```python
from build123d import *

# Parameters (mm, degrees)
SKETCH1_R           = 1.6383
SKETCH1_R_2         = 0.8382
BOSS_EXTRUDE1_DEPTH = 1.575


with BuildPart() as part:
    # Sketch1 → Boss-Extrude1 (new body)
    with BuildSketch(Plane(origin=(0, 0, 0), x_dir=(1, 0, 0), z_dir=(0, 1, 0))):
        with BuildLine():
            Line((-38.39500299, 29.999999735), (-42.73000299, 29.999999735))
            Line((-42.73000299, 29.999999735), (-44.000003042, 30.013999735))
            Line((-44.000003042, 30.013999735), (-44.000003042, 31.269999735))
            Line((-44.000003042, 31.269999735), (-44.00000361, 44.999999735))
            ThreePointArc((-44.00000361, 44.999999735), (-43.414217128, 46.414213903), (-42.000002924, 47.000000297))
            Line((-42.000002924, 47.000000297), (-30.435003745, 47.000000297))
            Line((-30.435003745, 47.000000297), (-30.435002721, 22.255354587))
            Line((-30.435002721, 22.255354587), (-11.909002721, 22.255355354))
            Line((-11.909002721, 22.255355354), (-11.909002721, -8.5))
            Line((-11.909002721, -8.5), (-23.409001447, -8.5))
            Line((-23.409001447, -8.5), (-23.409000495, -31.499999412))
            Line((-23.409000495, -31.499999412), (23.408999505, -31.499997474))
            Line((23.408999505, -31.499997474), (23.408999505, -8.499997555))
            Line((23.408999505, -8.499997555), (11.908997279, -8.499997555))
            Line((11.908997279, -8.499997555), (11.908997279, 22.25535634))
            Line((11.908997279, 22.25535634), (30.434997279, 22.255357107))
            Line((30.434997279, 22.255357107), (30.434996255, 47.000002817))
            Line((30.434996255, 47.000002817), (41.999997246, 47.000002817))
            ThreePointArc((41.999997246, 47.000002817), (43.414210615, 46.414216484), (43.999996958, 45.000003119))
            Line((43.999996958, 45.000003119), (43.999996958, 32.000003378))
            Line((43.999996958, 32.000003378), (43.999996958, 30.014003378))
            Line((43.999996958, 30.014003378), (32.823996958, 30.032002916))
            Line((32.823996958, 30.032002916), (32.823999503, -31.453997084))
            Line((32.823999503, -31.453997084), (36.099999555, -31.453996949))
            Line((36.099999555, -31.453996949), (36.099999785, -36.999996949))
            Line((36.099999785, -36.999996949), (43.849731264, -36.999996949))
            Line((43.849731264, -36.999996949), (43.849731264, -46.999996628))
            Line((43.849731264, -46.999996628), (-42.000000215, -46.999996628))
            ThreePointArc((-42.000000215, -46.999996628), (-43.414212607, -46.414211361), (-44.000000215, -44.999999938))
            Line((-44.000000215, -44.999999938), (-44.000000215, -38.976999938))
            ThreePointArc((-44.000000215, -38.976999938), (-43.409460005, -37.574276579), (-42.000000215, -36.999999938))
            Line((-42.000000215, -36.999999938), (-38.395000215, -36.999999938))
            Line((-38.395000215, -36.999999938), (-36.100000319, -36.999999938))
            Line((-36.100000319, -36.999999938), (-36.100000549, -31.453999938))
            Line((-36.100000549, -31.453999938), (-32.824000497, -31.453999802))
            Line((-32.824000497, -31.453999802), (-32.824003042, 30.014000198))
            Line((-32.824003042, 30.014000198), (-38.39500299, 29.999999735))
        make_face()
        with Locations(Location((40, 43.5, 0), (0, 0, 270))):
            Circle(SKETCH1_R, mode=Mode.SUBTRACT)
        with Locations(Location((-40, 43.5, 0), (0, 0, 270))):
            Circle(SKETCH1_R, mode=Mode.SUBTRACT)
        with Locations(Location((-37.6, -42.2, 0), (0, 0, 270))):
            Circle(SKETCH1_R, mode=Mode.SUBTRACT)
        with Locations(Location((36.1, -42.2, 0), (0, 0, 270))):
            Circle(SKETCH1_R, mode=Mode.SUBTRACT)
        with Locations(Location((-36.785003304, 36.350000034, 0), (0, 0, 270))):
            Circle(SKETCH1_R_2, mode=Mode.SUBTRACT)
        with Locations(Location((-26.220002542, 17.93192918, 0), (0, 0, 270))):
            Circle(SKETCH1_R_2, mode=Mode.SUBTRACT)
        with Locations(Location((26.219997458, 17.931931351, 0), (0, 0, 270))):
            Circle(SKETCH1_R_2, mode=Mode.SUBTRACT)
        with Locations(Location((36.784996695, 36.36800308, 0), (0, 0, 270))):
            Circle(SKETCH1_R_2, mode=Mode.SUBTRACT)
    extrude(amount=BOSS_EXTRUDE1_DEPTH)


solid = part.part
```
Verification items for the finished model (mm, model axes). Give positions to 0.01 mm unless a question says otherwise; leave off trailing zeros. Write each loop counter-clockwise with the first axis right and the second up, starting at its lowest first coordinate (ties: lowest second). Pieces come first, ordered by that corner, then holes. Notation, with made-up numbers: M -13,-22.75 L 32,-22.75 A15 ccw 32,-4.75 Z; hole C 82.25,-4.75 d11. An arc over 180 degrees is marked long. One line per question, with ' | ' between items.
1) Thickness scan on line 1 along X through (y, z) = (0.3, -43.5) (3 decimals); line 2 along X through (y, z) = (0.55, 42.2); line 3 along Z through (x, y) = (-17.5, 1.3). Record the ranges inside material, lowest first. Write a range as [from, to].
Result:
line 1: x = [-44, -41.638], [-38.362, -30.435], [30.435, 38.362], [41.638, 44] | line 2: x = [-44, -39.24], [-35.96, 34.46], [37.74, 43.85] | line 3: z = [-22.26, 8.5], [31.5, 47]
2) Mould release check, pull along X, two halves, no side actions. Record for faces 1 (the cylindrical face through (-43.43, 0.78, -46.4)), 2 (the cylindrical face through (43.4, 0.78, -46.43)), 3 (the cylindrical face through (-39.2, 0.78, 41.84)), 4 (the cylindrical face through (-38.62, 0.78, -42.62)): released by +X, released by -X, zero draft, split by the parting line, or undercut.
Result:
face 1: released by -X | face 2: released by +X | face 3: undercut | face 4: undercut
3) Section check C-C on z = -4.5. Enter the section's corners in (x, y) (3 decimals).
Result:
outline: M -32.824,0 L -11.909,0 L -11.909,1.575 L -32.824,1.575 Z; M 11.909,0 L 32.824,0 L 32.824,1.575 L 11.909,1.575 Z
4) Section check B-B on x = 18. Enter the section's corners in (y, z) (3 decimals), plus the area to 3 significant figures.
Result:
outline: M 0,-22.255 L 1.575,-22.255 L 1.575,8.5 L 0,8.5 Z; M 0,31.5 L 1.575,31.5 L 1.575,47 L 0,47 Z | area: 72.9 mm2
5) Section check D-D on x = 40. Enter the section's corners in (y, z) (3 decimals).
Result:
outline: M 0,-47 L 1.575,-47 L 1.575,-45.138 L 0,-45.138 Z; M 0,-41.862 L 1.575,-41.862 L 1.575,-30.02 L 0,-30.02 Z; M 0,37 L 1.575,37 L 1.575,47 L 0,47 Z
6) Gauge pin test, flat ends, axial feed: pin 1 Ø1.9 at (x, z) = (36.78, -36.37) entering from -Y; pin 2 Ø0.5 at (y, z) = (1, -2) entering from -X. Record the tip position at first contact, or that the pin passes through.
Result:
pin 1: stops at y = 0 | pin 2: stops at x = -32.82
7) Section check A-A on z = 42.2. Enter the section's corners in (x, y) (3 decimals), plus the area to 3 significant figures.
Result:
outline: M -44,0 L -39.238,0 L -39.238,1.575 L -44,1.575 Z; M -35.962,0 L 34.462,0 L 34.462,1.575 L -35.962,1.575 Z; M 37.738,0 L 43.85,0 L 43.85,1.575 L 37.738,1.575 Z | area: 128 mm2
